Geometry check sheet. Reference: drawing and pictorial views, mm from the part's lowest x, y, z. Coordinates: 2 decimals unless noted, no trailing zeros. Write each loop counter-clockwise with the first axis right and the second up, starting at its lowest first coordinate (ties: lowest second). Pieces come first, ordered by that corner, then holes. Notation, with made-up numbers: (74.25, 87) -> (127.25, 87) arc R14 cw to (127.25, 91) -> close; hole circle Ø5 at (24, 62). An arc over 180 degrees is marked (long way). Use a Markdown table: item, result.
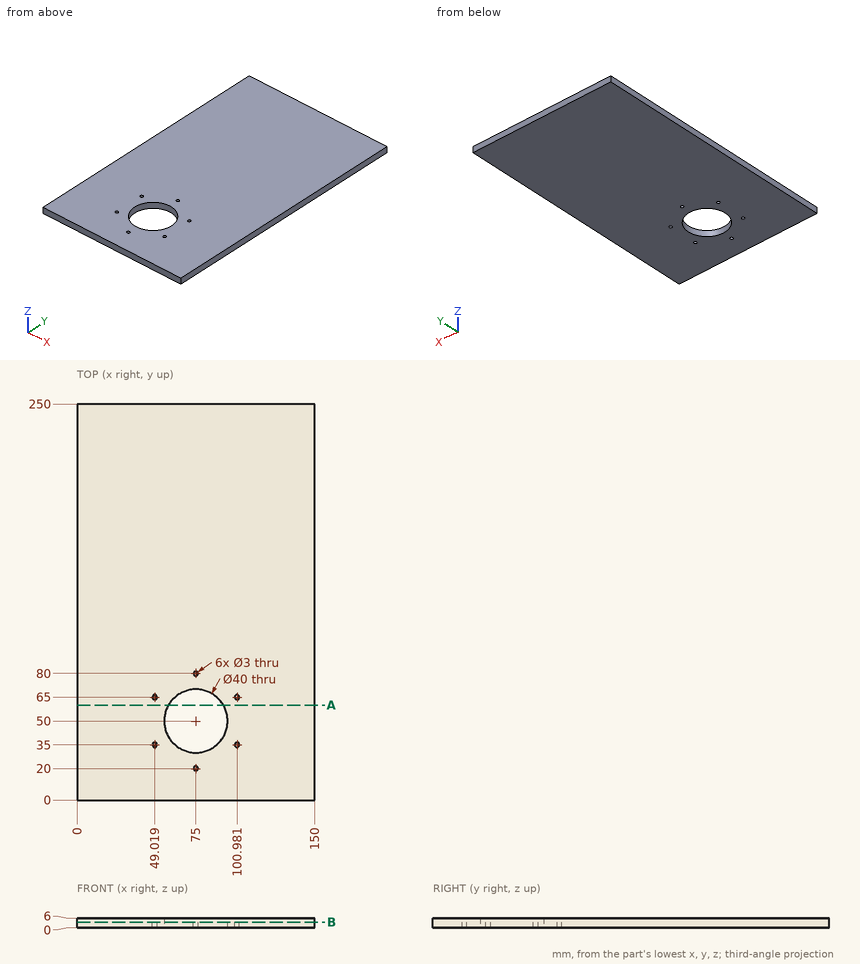
Item 1: Depth check by flat-ended pin: P1, Ø24, axis at x = 75, y = 50, coming from the -Z side; P2, Ø4, axis at x = 75, y = 80, coming from the -Z side. Enter the tip coordinate at first touch or a pass-through.
Answer block:
| item | result |
|---|---|
| P1 | passes through |
| P2 | stops at z = 0 |
Item 2: Thickness scan on L1, parallel to X at y = 65, z = 3.3; L2, parallel to X at y = 40.5, z = 5.05; L3, parallel to Y at x = 66, z = 2.1. Record the ranges inside material, lowest first. Write a range as [from, to].
Answer block:
| item | result |
|---|---|
| L1 | x = [0, 47.52], [50.52, 61.77], [88.23, 99.48], [102.48, 150] |
| L2 | x = [0, 57.4], [92.6, 150] |
| L3 | y = [0, 32.14], [67.86, 250] |
Item 3: Section check A-A on y = 60. Record the boundary of the cut face in (x, z), then the cut area to 3 significant figures.
Answer block:
| item | result |
|---|---|
| outline | (0, 0) -> (57.68, 0) -> (57.68, 6) -> (0, 6) -> close; (92.32, 0) -> (150, 0) -> (150, 6) -> (92.32, 6) -> close |
| area | 692 mm^2 |
Item 4: Section check B-B on z = 3.5. Record the boundary of the cut face in (x, y), then the cut area to 3 significant figures.
Answer block:
| item | result |
|---|---|
| outline | (0, 0) -> (150, 0) -> (150, 250) -> (0, 250) -> close; hole circle Ø3 at (49.02, 35); hole circle Ø3 at (49.02, 65); hole circle Ø40 at (75, 50); hole circle Ø3 at (75, 20); hole circle Ø3 at (75, 80); hole circle Ø3 at (100.98, 35); hole circle Ø3 at (100.98, 65) |
| area | 36,200 mm^2 |
